```python
from build123d import *

# Parameters (mm, degrees)
F1_DEPTH = 2
F2_DEPTH = 5.6506898254
F3_DEPTH = 3


with BuildPart() as f1:
    # F0 (on Top) → F1 (new body)
    with BuildSketch(Plane.XY):
        Polygon((-43.2085677565, 22.6745967576), (-58.8549531333, -4.4257376699), (-38.4300476107, -4.4257376699), (-40.2088151152, 5.6621541398), (-48.0090622621, 5.6621541398), (-48.5864125313, 6.6621541398), (-48.0090622621, 7.6621541398), (-40.5614690766, 7.6621541398), align=None)
    extrude(amount=F1_DEPTH)



with BuildPart() as f1b:
    # F0 (on Top) → F1, piece 2 (new body)
    with BuildSketch(Plane.XY):
        Polygon((-41.2085677565, 22.6745967576), (-36.4300476107, -4.4257376699), (-25.5239465254, -4.4257376699), (-23.5239465254, -4.4257376699), (-23.1770010553, -4.4257376699), (-25.5239465254, 8.8844515061), (-33.4898163741, 8.8844515061), (-34.0671666433, 9.8844515061), (-33.4898163741, 10.8844515061), (-22.7936475677, 10.8844515061), (-20.0940481363, -4.4257376699), (-3.2846095154, -4.4257376699), (4.538583173, 9.1244295439), (-3.2846095154, 22.6745967576), (-20.0940481363, 22.6745967576), (-24.4790815038, 15.0794961721), (-25.6024042349, 14.7936511306), (-33.2868439501, 22.6745967576), align=None)
        Polygon((-15.4996355878, 9.1244295439), (-13.5944822068, 12.424251996), (-9.7841754448, 12.424251996), (-7.8790220638, 9.1244295439), (-9.7841754448, 5.8246070917), (-13.5944822068, 5.8246070917), align=None, mode=Mode.SUBTRACT)
    extrude(amount=F1_DEPTH)


with BuildPart() as f1_1:
    add(f1.part)

    add(f1b.part)  # F2 merges F1b
    # F0 (on Top) → F2 (join)
    with BuildSketch(Plane.XY):
        Polygon((-20.0940481363, 24.6745967576), (-44.3632682949, 24.6745967576), (-62.3190547484, -6.4257376699), (-38.9180315569, -6.4257376699), (-2.129908977, -6.4257376699), (6.8479842498, 9.1244295439), (6.2706339806, 10.1244295439), (-2.129908977, 24.6745967576), (-2.8602079346, 24.6745967576), align=None)
        Polygon((-38.4300476107, -4.4257376699), (-58.8549531333, -4.4257376699), (-43.2085677565, 22.6745967576), (-41.2085677565, 22.6745967576), (-33.2868439501, 22.6745967576), (-30.5356123181, 22.6745967576), (-20.0940481363, 22.6745967576), (-3.2846095154, 22.6745967576), (4.538583173, 9.1244295439), (-3.2846095154, -4.4257376699), (-20.0940481363, -4.4257376699), (-23.1770010553, -4.4257376699), (-23.5239465254, -4.4257376699), (-25.5239465254, -4.4257376699), (-36.4300476107, -4.4257376699), align=None, mode=Mode.SUBTRACT)
        Polygon((-41.2085677565, 22.6745967576), (-36.4300476107, -4.4257376699), (-25.5239465254, -4.4257376699), (-23.5239465254, -4.4257376699), (-23.1770010553, -4.4257376699), (-25.5239465254, 8.8844515061), (-33.4898163741, 8.8844515061), (-34.0671666433, 9.8844515061), (-33.4898163741, 10.8844515061), (-22.7936475677, 10.8844515061), (-20.0940481363, -4.4257376699), (-3.2846095154, -4.4257376699), (4.538583173, 9.1244295439), (-3.2846095154, 22.6745967576), (-20.0940481363, 22.6745967576), (-24.4790815038, 15.0794961721), (-25.6024042349, 14.7936511306), (-33.2868439501, 22.6745967576), align=None)
        Polygon((-15.4996355878, 9.1244295439), (-13.5944822068, 12.424251996), (-9.7841754448, 12.424251996), (-7.8790220638, 9.1244295439), (-9.7841754448, 5.8246070917), (-13.5944822068, 5.8246070917), align=None, mode=Mode.SUBTRACT)
        Polygon((-25.5239465254, 8.8844515061), (-23.1770010553, -4.4257376699), (-20.0940481363, -4.4257376699), (-22.7936475677, 10.8844515061), (-33.4898163741, 10.8844515061), (-34.0671666433, 9.8844515061), (-33.4898163741, 8.8844515061), align=None)
        Polygon((-40.2088151152, 5.6621541398), (-38.4300476107, -4.4257376699), (-36.4300476107, -4.4257376699), (-41.2085677565, 22.6745967576), (-43.2085677565, 22.6745967576), (-40.5614690766, 7.6621541398), align=None)
        Polygon((-20.0940481363, 22.6745967576), (-30.5356123181, 22.6745967576), (-24.1704509766, 16.1898996279), (-24.4790815038, 15.0794961721), align=None)
        Polygon((-30.5356123181, 22.6745967576), (-33.2868439501, 22.6745967576), (-25.6024042349, 14.7936511306), (-24.4790815038, 15.0794961721), (-24.1704509766, 16.1898996279), align=None)
        Polygon((-48.0090622621, 5.6621541398), (-40.2088151152, 5.6621541398), (-40.5614690766, 7.6621541398), (-48.0090622621, 7.6621541398), (-48.5864125313, 6.6621541398), align=None)
    extrude(amount=F2_DEPTH)

    # F0 (on Top) → F3 (join)
    with BuildSketch(Plane.XY):
        Polygon((-9.7841754448, 12.424251996), (-13.5944822068, 12.424251996), (-15.4996355878, 9.1244295439), (-13.5944822068, 5.8246070917), (-9.7841754448, 5.8246070917), (-7.8790220638, 9.1244295439), align=None)
    extrude(amount=F3_DEPTH)


solid = f1_1.part
```
Check sheet for the modelled part. Datum: model origin and axes. Units: mm. A direction names the side the tool comes from. Coordinates: 2 decimals unless noted, no trailing zeros. Order: outer loops, then holes, each group sorted by start corner. A loop starts at its lowest first (then second) coordinate and runs counter-clockwise, first axis right, second up. Notation, with made-up numbers: (9, 46.25) -> (54, 46.25) arc R17 ccw to (54, 61.25) -> close; hole circle Ø3 at (60, 3.25). An arc over 180 degrees is marked (long way). Write each question's results on one line, items separated by ' | '. Start each with the question number.
1) Set-up check for faces 1 (the face through (-33, -6.426, 3)), 2 (the face through (-48, -4.426, 4)): record each of +Z, -Z, +X, -X, +Y, -Y from which the full face is reachable in a straight line by a thin tool's end or side.
2) Section check D-D (y = 15). Enter the section's corners in (x, z), and give its area (3 significant figures).
3) Draft check along X on faces 3 (the face through (-21, 9, 5.651)), 4 (the face through (-53.215, 9.342, 2.786)), 5 (the face through (-41.904, 15.273, 3.8)). Enter one of: pulls with the +X half, pulls with the -X half, needs draft (parallel to the pull), parting line crosses it, or undercut.
4) Section check C-C (x = -58). Enter the section's corners in (y, z).
5) Material ranges on line 1 along X through (y, z) = (11.5, 4); line 2 along Y through (x, z) = (-11, 3.75); line 3 along X through (y, z) = (1, 4.3), recorded low to high.
6) Depth check by flat-ended pin: pin 1 (3 mm diameter, centred on x = -46, z = 4.5, fed in from +Y); pin 2 (3.5 mm diameter, centred on x = -13.5, y = 8, fed in from +Z). Enter the tip coordinate at first touch or a pass-through.
7) Section check A-A (z = 4.55). Enter the section's corners in (x, y), and give its area (3 significant figures).
8) Section check B-B (z = 1.35). Enter the section's corners in (x, y).
Checked values:
1) face 1: +Z, -Z, +X, -X, -Y | face 2: +Z
2) outline: (-49.95, 0) -> (3.46, 0) -> (3.46, 5.65) -> (-41.86, 5.65) -> (-41.86, 2) -> (-47.64, 2) -> (-47.64, 5.65) -> (-49.95, 5.65) -> close | area: 281 mm²
3) face 3: needs draft | face 4: pulls with the -X half | face 5: undercut
4) outline: (-6.43, 0) -> (1.06, 0) -> (1.06, 5.65) -> (-2.94, 5.65) -> (-2.94, 2) -> (-4.43, 2) -> (-4.43, 5.65) -> (-6.43, 5.65) -> close
5) line 1: -51.97 to -49.66, -41.24 to -14.13, -9.25 to 5.48 | line 2: -6.43 to 5.82, 12.42 to 24.67 | line 3: -58.03 to -55.72, -39.39 to 2.16
6) pin 1: y = 24.44 | pin 2: z = 5.65
7) outline: (-62.32, -6.43) -> (-2.13, -6.43) -> (6.85, 9.12) -> (-2.13, 24.67) -> (-44.36, 24.67) -> close; hole (-58.85, -4.43) -> (-38.43, -4.43) -> (-40.21, 5.66) -> (-48.01, 5.66) -> (-48.59, 6.66) -> (-48.01, 7.66) -> (-40.56, 7.66) -> (-43.21, 22.67) -> close; hole (-15.5, 9.12) -> (-13.59, 5.82) -> (-9.78, 5.82) -> (-7.88, 9.12) -> (-9.78, 12.42) -> (-13.59, 12.42) -> close | area: 1,430 mm²
8) outline: (-62.32, -6.43) -> (-2.13, -6.43) -> (6.85, 9.12) -> (-2.13, 24.67) -> (-44.36, 24.67) -> close
